```python
from build123d import *

# Parameters (mm, degrees)
SKETCH1_R           = 67.5
BOSS_EXTRUDE1_DEPTH = 25
SKETCH2_R           = 7.5
CUT_EXTRUDE1_DEPTH  = 99.67877178
SKETCH3_R           = 9.726631354
CUT_EXTRUDE2_DEPTH  = 15.23068
CIRPATTERN1_START   = 9.76931969
CIRPATTERN1_DEPTH   = 15.23068031


# Read off the part's stored shape, not the designer's step: CirPattern1
with BuildPart() as part:
    # Sketch1 → Boss-Extrude1 (new body)
    with BuildSketch(Plane(origin=(0, 0, 0), x_dir=(1, 0, 0), z_dir=(0, 1, 0))):
        with Locations(Location((0, 0, 0), (0, 0, 270))):
            Circle(SKETCH1_R)
    extrude(amount=BOSS_EXTRUDE1_DEPTH)

    # Sketch2 → Cut-Extrude1 (cut, through all)
    with BuildSketch(Plane(origin=(0, 0, 0), x_dir=(1, 0, 0), z_dir=(0, 1, 0))):
        with Locations(Location((0, 0, 0), (0, 0, 270))):
            Circle(SKETCH2_R)
    extrude(amount=CUT_EXTRUDE1_DEPTH, mode=Mode.SUBTRACT)

    # Sketch3 → Cut-Extrude2 (cut)
    with BuildSketch(Plane(origin=(0, 25, 0), x_dir=(1, 0, 0), z_dir=(0, 1, 0))):
        with Locations(Location((-25.223681721, 0, 0), (0, 0, 270))):
            Circle(SKETCH3_R)
    extrude(amount=-CUT_EXTRUDE2_DEPTH, mode=Mode.SUBTRACT)

    # CirPattern1 outline → CirPattern1 (cut)
    with BuildSketch(Plane(origin=(0, 0, 0), x_dir=(1, 0, 0), z_dir=(0, 1, 0)).offset(CIRPATTERN1_START)):
        with BuildLine():
            ThreePointArc((8.459811138, -20.423790784), (0, -15.497050367), (-8.459811138, -20.423790784))
            ThreePointArc((-8.459811138, -20.423790784), (-10.958069403, -10.958069403), (-20.423790784, -8.459811138))
            ThreePointArc((-20.423790784, -8.459811138), (-21.501461049, -8.986235628), (-22.635727329, -9.376025254))
            ThreePointArc((-22.635727329, -9.376025254), (-24.71360338, -24.71360338), (-9.376025254, -22.635727329))
            ThreePointArc((-9.376025254, -22.635727329), (0, -34.950313075), (9.376025254, -22.635727329))
            ThreePointArc((9.376025254, -22.635727329), (24.71360338, -24.71360338), (22.635727329, -9.376025254))
            ThreePointArc((22.635727329, -9.376025254), (34.950313075, 0), (22.635727329, 9.376025254))
            ThreePointArc((22.635727329, 9.376025254), (24.71360338, 24.71360338), (9.376025254, 22.635727329))
            ThreePointArc((9.376025254, 22.635727329), (0, 34.950313075), (-9.376025254, 22.635727329))
            ThreePointArc((-9.376025254, 22.635727329), (-24.71360338, 24.71360338), (-22.635727329, 9.376025254))
            ThreePointArc((-22.635727329, 9.376025254), (-21.501461049, 8.986235628), (-20.423790784, 8.459811138))
            ThreePointArc((-20.423790784, 8.459811138), (-10.958069403, 10.958069403), (-8.459811138, 20.423790784))
            ThreePointArc((-8.459811138, 20.423790784), (0, 15.497050367), (8.459811138, 20.423790784))
            ThreePointArc((8.459811138, 20.423790784), (10.958069403, 10.958069403), (20.423790784, 8.459811138))
            ThreePointArc((20.423790784, 8.459811138), (15.497050367, 0), (20.423790784, -8.459811138))
            ThreePointArc((20.423790784, -8.459811138), (10.958069403, -10.958069403), (8.459811138, -20.423790784))
        make_face()
    extrude(amount=CIRPATTERN1_DEPTH, mode=Mode.SUBTRACT)


solid = part.part
```
The listing builds one solid part. Answer for the finished solid, in the listing's coordinates (mm). A direction names the side the tool comes from. Coordinates: 2 decimals unless noted, no trailing zeros. Write each loop counter-clockwise with the first axis right and the second up, starting at its lowest first coordinate (ties: lowest second). Pieces come first, ordered by that corner, then holes.
Q1. Section B-B, the plane y = 19.25 is taken. Write down the section's boundary in (x, z), then the cut area to 3 significant figures.
Returned:
outline: circle Ø135 at (0, 0); (-20.42, -8.46) arc R9.73 cw to (-8.46, -20.42) arc R9.73 cw to (8.46, -20.42) arc R9.73 cw to (20.42, -8.46) arc R9.73 cw to (20.42, 8.46) arc R9.73 cw to (8.46, 20.42) arc R9.73 cw to (-8.46, 20.42) arc R9.73 cw to (-20.42, 8.46) arc R9.73 cw to start; hole (-22.64, -9.38) arc R9.73 ccw (long way) to (-9.38, -22.64) arc R9.73 ccw (long way) to (9.38, -22.64) arc R9.73 ccw (long way) to (22.64, -9.38) arc R9.73 ccw (long way) to (22.64, 9.38) arc R9.73 ccw (long way) to (9.38, 22.64) arc R9.73 ccw (long way) to (-9.38, 22.64) arc R9.73 ccw (long way) to (-22.64, 9.38) arc R9.73 ccw (long way) to start; hole circle Ø15 at (0, 0)
area: 11,800 mm2
Q2. Which of the six approach directions +Z, -Z, +X, -X, +Y, -Y give full straight-line access (tool end or side, diameter ignored) to faces 4 (the flat face through (0, 25, 9)), 5 (the cylindrical face through (10.86, 17.28, -11.06))?
Returned:
face 4: +Z, -Z, +X, -X, +Y
face 5: +Y
Q3. Given P1, Ø5, axis at x = 19, z = -3, coming from the +Y side; P2, Ø1, axis at x = 38.5, y = 3.5, coming from the +Z side; P3, Ø2, axis at y = 9.5, z = -15, coming from the +X side; P4, Ø13.5, axis at x = 0, z = 0, coming from the +Y side, each flat-ended and moving along its own axis, determine where each tip first touches the part or whether it passes through.
Returned:
P1: stops at y = 9.77
P2: stops at z = 55.79
P3: stops at x = 66.03
P4: passes through
Q4. Section C-C, the plane x = 0 is taken. Write down the section's boundary in (y, z).
Returned:
outline: (0, -67.5) - (25, -67.5) - (25, -34.95) - (9.77, -34.95) - (9.77, -15.5) - (25, -15.5) - (25, -7.5) - (0, -7.5) - close; (0, 7.5) - (25, 7.5) - (25, 15.5) - (9.77, 15.5) - (9.77, 34.95) - (25, 34.95) - (25, 67.5) - (0, 67.5) - close
Q5. Section D-D, the plane y = 3 is taken. Write down the section's boundary in (x, z), then the cut area to 3 significant figures.
Returned:
outline: circle Ø135 at (0, 0); hole circle Ø15 at (0, 0)
area: 14,100 mm2
Q6. Find the intervals of material crossed by line 1 along X through (y, z) = (17.25, 0); line 2 along Z through (x, y) = (-19.5, 23); line 3 along X through (y, z) = (20, 11), in increasing order.
Returned:
line 1: x = -67.5 to -34.95, -15.5 to -7.5, 7.5 to 15.5, 34.95 to 67.5
line 2: z = -64.62 to -27.42, -8.25 to -7.86, 7.86 to 8.25, 27.42 to 64.62
line 3: x = -66.6 to -24.76, -10.92 to 10.92, 24.76 to 66.6
Q7. The mould has two halves that part along X. Classify faces 1 (the cylindrical face through (-59.884, 12.325, 31.147)), 2 (the flat face through (-14, 25, 29)), 3 (the cylindrical face through (-15.5, 17.49, 0.14)): released by +X, released by -X, zero draft, split by the parting line, or undercut.
Returned:
face 1: split by the parting line
face 2: zero draft
face 3: undercut
Q8. Section A-A, the plane z = 0 is taken. Write down the section's boundary in (x, y).
Returned:
outline: (-67.5, 0) - (-7.5, 0) - (-7.5, 25) - (-15.5, 25) - (-15.5, 9.77) - (-34.95, 9.77) - (-34.95, 25) - (-67.5, 25) - close; (7.5, 0) - (67.5, 0) - (67.5, 25) - (34.95, 25) - (34.95, 9.77) - (15.5, 9.77) - (15.5, 25) - (7.5, 25) - close
